from build123d import *

# Parameters (mm, degrees)
SKETCH2_W           = 70
SKETCH2_H           = 40
BOSS_EXTRUDE1_DEPTH = 1.3
SKETCH4_W           = 14
SKETCH4_H           = 1.3
BOSS_EXTRUDE3_DEPTH = 1.5
SKETCH8_W           = 12.5
SKETCH8_H           = 6
BOSS_EXTRUDE4_DEPTH = 6
SKETCH9_W           = 1
SKETCH9_H           = 2.3
BOSS_EXTRUDE5_DEPTH = 0.8
SKETCH6_W           = 19
SKETCH6_H           = 15.5
CUT_EXTRUDE1_DEPTH  = 1.3


with BuildPart() as part:
    # Sketch2 → Boss-Extrude1 (new body)
    with BuildSketch(Plane.XY):
        with Locations((35, 20)):
            Rectangle(SKETCH2_W, SKETCH2_H)
    extrude(amount=BOSS_EXTRUDE1_DEPTH)

    # Sketch4 → Boss-Extrude3 (add)
    with BuildSketch(Plane(origin=(0, 40, 0), x_dir=(1, 0, 0), z_dir=(0, 1, 0))):
        with Locations((63, -0.65)):
            Rectangle(SKETCH4_W, SKETCH4_H)
    extrude(amount=BOSS_EXTRUDE3_DEPTH)

    # Sketch8 → Boss-Extrude4 (add)
    with BuildSketch(Plane(origin=(0, 0, 0), x_dir=(-1, 0, 0), z_dir=(0, 0, -1))):
        with Locations((-63.75, 38.5)):
            Rectangle(SKETCH8_W, SKETCH8_H)
        with Locations((-63.75, 3)):
            Rectangle(SKETCH8_W, SKETCH8_H)
    extrude(amount=BOSS_EXTRUDE4_DEPTH)

    # Sketch9 → Boss-Extrude5 (add)
    with BuildSketch(Plane(origin=(0, 0, -6), x_dir=(-1, 0, 0), z_dir=(0, 0, -1))):
        with Locations((-66, 38.5)):
            Rectangle(SKETCH9_W, SKETCH9_H)
        with Locations((-66, 3)):
            Rectangle(SKETCH9_W, SKETCH9_H)
    extrude(amount=BOSS_EXTRUDE5_DEPTH)

    # Sketch6 → Cut-Extrude1 (cut)
    with BuildSketch(Plane.XY.offset(1.3)):
        with Locations((60.5, 20.75)):
            Rectangle(SKETCH6_W, SKETCH6_H)
    extrude(amount=-CUT_EXTRUDE1_DEPTH, mode=Mode.SUBTRACT)


solid = part.part
Can you work these out from the model? Positions are in its coordinate system, mm. A direction names the side the tool comes from. Round coordinates to 2 decimals unless told otherwise and drop trailing zeros. Order: outer loops, then holes, each group sorted by start corner. A loop starts at its lowest first (then second) coordinate and runs counter-clockwise, first axis right, second up. Notation, with made-up numbers: (32, -27) - (40, -27) arc R23 cw to (40, -1) - close; hole circle Ø3 at (-1, 0). An arc over 180 degrees is marked (long way). Answer in a Markdown table with one row per item.
(1) Suppose I cut it at D-D, the plane y = 5. Please give me the cut outline in (x, z), plus the area to 3 significant figures.
From the geometry:
| item | result |
|---|---|
| outline | (0, 0) - (57.5, 0) - (57.5, -6) - (70, -6) - (70, 1.3) - (0, 1.3) - close |
| area | 166 mm2 |
(2) Which directions (+Z, -Z, +X, -X, +Y, -Y) give clear straight access to the entire face, cutting with the end or side of a thin tool? Please do faces 4 (the face through (28, 40, 1)), 5 (the face through (51, 21, 1)), 6 (the face through (64, 6, -3)), 7 (the face through (57.5, 3, -3)), 8 (the face through (70, 4, -1)).
From the geometry:
| item | result |
|---|---|
| face 4 | +Z, -Z, -X, +Y |
| face 5 | +Z, -Z, +X |
| face 6 | -Z, +X, -X |
| face 7 | -Z, -X, +Y, -Y |
| face 8 | +Z, -Z, +X, +Y, -Y |
(3) Suppose I cut it at A-A, the plane z = -2. Please give me the cut outline in (x, y).
From the geometry:
| item | result |
|---|---|
| outline | (57.5, 0) - (70, 0) - (70, 6) - (57.5, 6) - close; (57.5, 35.5) - (70, 35.5) - (70, 41.5) - (57.5, 41.5) - close |
(4) Suppose I cut it at B-B, the plane x = 54. Please give me the cut outline in (y, z).
From the geometry:
| item | result |
|---|---|
| outline | (0, 0) - (13, 0) - (13, 1.3) - (0, 1.3) - close; (28.5, 0) - (40, 0) - (40, 1.3) - (28.5, 1.3) - close |
(5) For P1, Ø12, axis at x = 30.5, y = 29.5, coming from the -Z side; P2, Ø3, axis at y = 3, z = -4, coming from the -X side; P3, Ø0.6, axis at x = 39.5, z = 0.5, coming from the +Y side, each with a flat end and sliding along its axis, tell me the tip position at first contact or that it passes through.
From the geometry:
| item | result |
|---|---|
| P1 | stops at z = 0 |
| P2 | stops at x = 57.5 |
| P3 | stops at y = 40 |
(6) If we mould it in two halves opening along Y, with no side actions, what happens to faces 1 (the face through (64, 35.5, -3)), 2 (the face through (63, 41.5, -2)), 3 (the face through (35, 20, 1.3))? For each: released by +Y, released by -Y, zero draft, split by the parting line, or undercut.
From the geometry:
| item | result |
|---|---|
| face 1 | undercut |
| face 2 | released by +Y |
| face 3 | zero draft |
(7) Suppose I cut it at C-C, the plane y = 38.5. Please give me the cut outline in (x, z).
From the geometry:
| item | result |
|---|---|
| outline | (0, 0) - (57.5, 0) - (57.5, -6) - (65.5, -6) - (65.5, -6.8) - (66.5, -6.8) - (66.5, -6) - (70, -6) - (70, 1.3) - (0, 1.3) - close |
(8) Please list where these lines run through material, in increasing order: L1, parallel to Y at x = 64, z = -3.75; L2, parallel to Z at x = 51, y = 38; L3, parallel to X at y = 20, z = 0.75. Write a range as from..to.
From the geometry:
| item | result |
|---|---|
| L1 | y = 0..6, 35.5..41.5 |
| L2 | z = 0..1.3 |
| L3 | x = 0..51 |
